Answer from the drawing. Dimensions are ordinates in mm from the lowest x, y and z of the part. A direction names the side the tool comes from. Give positions to 0.01 mm unless a question says otherwise; leave off trailing zeros. Loops run counter-clockwise (first coordinate to the right, second up) from the corner with the lowest first, then second, coordinate; pieces in that order, holes last. Notation, with made-up numbers: (15, 52.5) - (59, 52.5) arc R18 cw to (59, 85.5) - close; hole circle Ø7 at (57.25, 83). An arc over 180 degrees is marked (long way). Answer as CSV lines item,"result". Start each with the question number.
1) Flat-ended cylindrical pins translate along their axes: pin 1 (1.5 mm diameter, centred on y = 23.5, z = 5, fed in from +X); pin 2 (4 mm diameter, centred on x = 25.5, z = 2.5, fed in from -Y). Find the tip coordinate at first contact, or state that the pin passes through.
2) For a pull along X with two mould halves and no side action, classify the marked faces 1 and 2 as pulls with the +X half, pulls with the -X half, needs draft (parallel to the pull), parting line crosses it, or undercut.
3) Find the intervals of material crossed by line 1 along Y through (x, z) = (10.5, 5.5); line 2 along X through (y, z) = (9.5, 6); line 3 along Y through (x, z) = (28.5, 4.5), in increasing order.
4) For the marked faces 3, 4 and 5, determine the directions among +Z, -Z, +X, -X, +Y, -Y from which every point of the face is accessible in a straight line to the end or side of a thin tool.
5) A cutting plane is placed at C-C (x = 29.5). Determine the outline of the cut face in (y, z).
6) A cutting plane is placed at B-B (z = 5.75). Determine the outline of the cut face in (x, y).
7) A cutting plane is placed at A-A (x = 15). Determine the outline of the cut face in (y, z).
8) A cutting plane is placed at D-D (y = 32.5). Determine the outline of the cut face in (x, z).
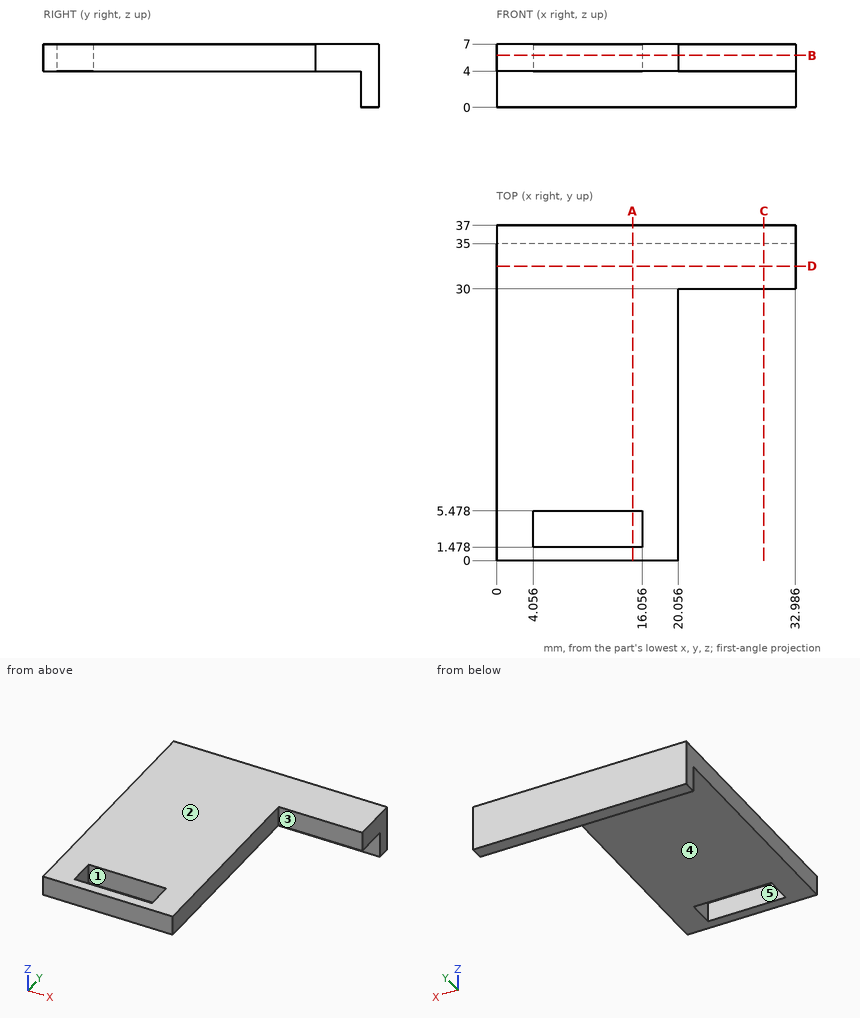
Ans:
1,pin 1,"x = 20.06"
1,pin 2,"y = 30"
2,face 1,"undercut"
2,face 2,"needs draft"
3,line 1,"0 to 1.48, 5.48 to 37"
3,line 2,"0 to 20.06"
3,line 3,"30 to 37"
4,face 3,"+Z, -Z, +X, -Y"
4,face 4,"-Z, +X, -X, -Y"
4,face 5,"+Z, -Z"
5,outline,"(30, 4) - (35, 4) - (35, 0) - (37, 0) - (37, 7) - (30, 7) - close"
6,outline,"(0, 0) - (20.06, 0) - (20.06, 30) - (32.99, 30) - (32.99, 37) - (0, 37) - close; hole (4.06, 1.48) - (16.06, 1.48) - (16.06, 5.48) - (4.06, 5.48) - close"
7,outline,"(0, 4) - (1.48, 4) - (1.48, 7) - (0, 7) - close; (5.48, 4) - (35, 4) - (35, 0) - (37, 0) - (37, 7) - (5.48, 7) - close"
8,outline,"(0, 4) - (32.99, 4) - (32.99, 7) - (0, 7) - close"
